Part model, mm, in its own coordinate system. Face numbers are marked on the shaded views. A direction names the side the tool comes from. Give positions to 0.01 mm unless a question says otherwise; leave off trailing zeros. Write each loop counter-clockwise with the first axis right and the second up, starting at its lowest first coordinate (ties: lowest second). Pieces come first, ordered by that corner, then holes. Notation, with made-up numbers: M 75,-37.5 L 106,-37.5 A17 cw 106,-19.5 Z; hole C 10,-2 d3. An arc over 180 degrees is marked long. Use CSV: the item, a comma, the result in double quotes. Start each with the question number.
Item 1: Which spindle directions (+Z, -Z, +X, -X, +Y, -Y) get a long thin tool onto all of the face, cutting with end or side? Do the marked faces 4, 5, 6 and 7. Say none if no direction does.
Item 2: Cut at A-A (z = 9). List the corners of the cut face in (x, y), then the cut area to 3 significant figures.
Item 3: Cut at B-B (x = 8). List the corners of the cut face in (y, z), then the cut area to 3 significant figures.
Item 4: Cut at D-D (y = 2.5). List the corners of the cut face in (x, z), then the cut area to 4 significant figures.
Item 5: Pin check, flat tips, straight feed: pin 1 (1.6 mm diameter, centred on x = 10.5, y = 8.5, fed in from -Z); pin 2 (3.5 mm diameter, centred on x = 8.5, y = -4, fed in from +Z); pin 3 (4 mm diameter, centred on x = 4.5, y = 6.5, fed in from +Z). Stop position of each tip, or through.
Item 6: Drill centre lines: line 1 (Y direction, x = 10.5, z = -3.75); line 2 (Y direction, x = 2.25, z = 4.5); line 3 (X direction, y = 2.5, z = 9.25). Where is each one in solid material? Low to high. Write a range as [from, to].
Item 7: Mould opens along Y. For the marked faces 1, 2 and 3 say: released by +Y, released by -Y, zero draft, split by the parting line, or undercut.
Item 8: Cut at C-C (z = -6). List the corners of the cut face in (x, y), then the cut area to 4 significant figures.
from build123d import *

# Parameters (mm, degrees)
ESQUISSE1_W             = 11.5
ESQUISSE1_H             = 9.8
BOSS_EXTRU_1_DEPTH      = 11
ESQUISSE2_W             = 9.5
ESQUISSE2_H             = 7.8
ENL_V_MAT_EXTRU_1_DEPTH = 10
ESQUISSE3_W             = 7.5
ESQUISSE3_H             = 3
ENL_V_MAT_EXTRU_2_DEPTH = 2.5
CONG_1_R                = 0.75
ESQUISSE4_W             = 11.5
ESQUISSE4_H             = 14.8
BOSS_EXTRU_2_DEPTH      = 1.5
ESQUISSE5_W             = 11.5
ESQUISSE5_H             = 1.25
BOSS_EXTRU_3_DEPTH      = 8
CONG_2_R                = 0.5
CONG_3_R                = 0.5


with BuildPart() as part:
    # Esquisse1 → Boss.-Extru.1 (new body)
    with BuildSketch(Plane.XY):
        with Locations((5.75, 4.9)):
            Rectangle(ESQUISSE1_W, ESQUISSE1_H)
    extrude(amount=BOSS_EXTRU_1_DEPTH)

    # Esquisse2 → Enlèv. mat.-Extru.1 (cut)
    with BuildSketch(Plane.XY.offset(11)):
        with Locations((5.75, 4.9)):
            Rectangle(ESQUISSE2_W, ESQUISSE2_H)
    extrude(amount=-ENL_V_MAT_EXTRU_1_DEPTH, mode=Mode.SUBTRACT)

    # Esquisse3 → Enlèv. mat.-Extru.2 (cut)
    with BuildSketch(Plane(origin=(0, 9.8, 0), x_dir=(1, 0, 0), z_dir=(0, 1, 0))):
        with Locations((5.75, -1.5)):
            Rectangle(ESQUISSE3_W, ESQUISSE3_H)
    extrude(amount=-ENL_V_MAT_EXTRU_2_DEPTH, mode=Mode.SUBTRACT)

    # Congé1
    cong_1_edges = [part.edges().sort_by_distance(p)[0] for p in [
        (5.75, 7.3, 1),
        (5.75, 8.8, 3),
    ]]
    fillet(cong_1_edges, radius=CONG_1_R)

    # Esquisse4 → Boss.-Extru.2 (add)
    with BuildSketch(Plane(origin=(0, 0, 0), x_dir=(-1, 0, 0), z_dir=(0, 0, -1))):
        with Locations((-5.75, -0.1)):
            Rectangle(ESQUISSE4_W, ESQUISSE4_H)
    extrude(amount=BOSS_EXTRU_2_DEPTH)

    # Esquisse5 → Boss.-Extru.3 (add)
    with BuildSketch(Plane(origin=(0, 0, -1.5), x_dir=(-1, 0, 0), z_dir=(0, 0, -1))):
        with Locations((-5.75, 6.675)):
            Rectangle(ESQUISSE5_W, ESQUISSE5_H)
        with Locations((-5.75, -6.875)):
            Rectangle(ESQUISSE5_W, ESQUISSE5_H)
    extrude(amount=BOSS_EXTRU_3_DEPTH)

    # Congé2
    cong_2_edges = [part.edges().sort_by_distance(p)[0] for p in [
        (5.75, -7.5, 0),
    ]]
    fillet(cong_2_edges, radius=CONG_2_R)

    # Congé3
    cong_3_edges = [part.edges().sort_by_distance(p)[0] for p in [
        (1, 9.8, 0),
        (10.5, 9.8, 0),
        (1, 7.3, 0),
    ]]
    fillet(cong_3_edges, radius=CONG_3_R)


solid = part.part
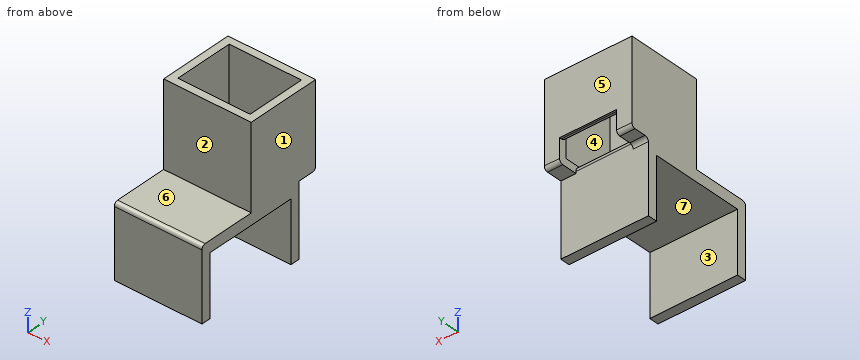
Worked answers:
1,face 4,"+Z"
1,face 5,"+Z, -Z, +X, -X, +Y"
1,face 6,"+Z, +X, -X, -Y"
1,face 7,"-Z, +X, -X"
2,outline,"M 0,0 L 11.5,0 L 11.5,9.8 L 0,9.8 Z; hole M 1,1 L 10.5,1 L 10.5,8.8 L 1,8.8 Z"
2,area,"38.6 mm^2"
3,outline,"M -7.5,-9.5 L -6.25,-9.5 L -6.25,-1.5 L 6.05,-1.5 L 6.05,-9.5 L 7.3,-9.5 L 7.3,0.25 A0.75 ccw 6.55,1 L 1,1 L 1,11 L 0,11 L 0,0 L -7,0 A0.5 ccw -7.5,-0.5 Z; M 8.8,3.75 A0.75 ccw 9.55,3 L 9.8,3 L 9.8,11 L 8.8,11 Z"
3,area,"67.2 mm^2"
4,outline,"M 0,-1.5 L 11.5,-1.5 L 11.5,11 L 10.5,11 L 10.5,1 L 1,1 L 1,11 L 0,11 Z"
4,area,"48.75 mm^2"
5,pin 1,"stops at z = 0"
5,pin 2,"stops at z = 0"
5,pin 3,"stops at z = 1"
6,line 1,"y = [-7.5, -6.25], [6.05, 7.3]"
6,line 2,"y = [0, 1], [8.8, 9.8]"
6,line 3,"x = [0, 1], [10.5, 11.5]"
7,face 1,"zero draft"
7,face 2,"released by -Y"
7,face 3,"undercut"
8,outline,"M 0,-7.5 L 11.5,-7.5 L 11.5,-6.25 L 0,-6.25 Z; M 0,6.05 L 11.5,6.05 L 11.5,7.3 L 0,7.3 Z"
8,area,"28.75 mm^2"
